```python
from build123d import *

# Parameters (mm, degrees)
CROQUIS1_W              = 8
CROQUIS1_H              = 15
SALIENTE_EXTRUIR6_DEPTH = 1.1
SALIENTE_EXTRUIR7_DEPTH = 2


with BuildPart() as part:
    # Croquis1 → Saliente-Extruir6 (new body)
    with BuildSketch(Plane.XY):
        Rectangle(CROQUIS1_W, CROQUIS1_H)
    extrude(amount=SALIENTE_EXTRUIR6_DEPTH)

    # Croquis8 → Saliente-Extruir7 (add, symmetric)
    with BuildSketch(Plane(origin=(0, 0, 0), x_dir=(0, 0, -1), z_dir=(1, 0, 0))):
        with BuildLine():
            Line((0, 7), (0, 5))
            ThreePointArc((0, 5), (5, 0), (0, -5))
            Line((0, -5), (0, -7))
            ThreePointArc((0, -7), (7, 0), (0, 7))
        make_face()
    extrude(amount=SALIENTE_EXTRUIR7_DEPTH, both=True)


solid = part.part
```
CAD build for the part. Positions are in the model's coordinates, mm. A direction names the side the tool comes from. Round coordinates to 2 decimals unless told otherwise and drop trailing zeros. Order: outer loops, then holes, each group sorted by start corner. A loop starts at its lowest first (then second) coordinate and runs counter-clockwise, first axis right, second up. Notation, with made-up numbers: (48.5, 8.25) -> (80.5, 8.25) arc R22 ccw to (80.5, 24.25) -> close; hole circle Ø8 at (31.25, -24). An arc over 180 degrees is marked (long way). One line per question, with ' | ' between items.
Q1. Slice it at C-C (z = -3.25). Write the cut outline in (x, y), then the cut area to 3 significant figures.
Completed:
outline: (-2, -6.2) -> (2, -6.2) -> (2, -3.8) -> (-2, -3.8) -> close; (-2, 3.8) -> (2, 3.8) -> (2, 6.2) -> (-2, 6.2) -> close | area: 19.2 mm^2
Q2. Which spindle directions (+Z, -Z, +X, -X, +Y, -Y) get a long thin tool onto all of the face, cutting with end or side? Do faces 4 (the flat face through (-2, 2, -5)), 5 (the flat face through (-4, -0.1, 0.5)), 6 (the flat face through (-0.1, -7.5, 0.5)), 7 (the cylindrical face through (0, 0, -5)), 8 (the flat face through (2, 2, -5)). Say none if no direction does.
Completed:
face 4: -Z, -X, +Y, -Y | face 5: +Z, -Z, -X, +Y, -Y | face 6: +Z, -Z, +X, -X, -Y | face 7: +X, -X | face 8: -Z, +X, +Y, -Y
Q3. Two-plate mould, pull along Z, no slides. Class faces 1 (the flat face through (0, 0, 1.1)), 2 (the cylindrical face through (0, 0, -7)), 3 (the flat face through (0, 0, 0)): released by +Z, released by -Z, zero draft, split by the parting line, or undercut.
Completed:
face 1: released by +Z | face 2: released by -Z | face 3: undercut
Q4. Probe probe 1 along Z at (x, y) = (0, 0); probe 2 along X at (y, z) = (1.5, -5); probe 3 along Y at (x, z) = (1.5, -0.75). List the from-to ranges inside material, lowest first.
Completed:
probe 1: z = -7 to -5, 0 to 1.1 | probe 2: x = -2 to 2 | probe 3: y = -6.96 to -4.94, 4.94 to 6.96
Q5. Drop flat-ended pins along their axis: pin 1 (1.5 mm diameter, centred on x = 1.5, z = -5, fed in from -Y); pin 2 (1.5 mm diameter, centred on y = 2, z = -4, fed in from +X); pin 3 (4 mm diameter, centred on x = -1.5, y = 3.5, fed in from -Z). Give the stop position or say it passes through.
Completed:
pin 1: stops at y = -5.56 | pin 2: stops at x = 2 | pin 3: stops at z = -6.84
Q6. Slice it at A-A (x = 0). Write the cut outline in (y, z), then the cut area to 3 significant figures.
Completed:
outline: (-7.5, 0) -> (-7, 0) arc R7 ccw to (7, 0) -> (7.5, 0) -> (7.5, 1.1) -> (-7.5, 1.1) -> close; hole (-5, 0) arc R5 ccw to (5, 0) -> close | area: 54.2 mm^2
Q7. Slice it at B-B (y = 0). Write the cut outline in (x, z), then the cut area to 3 significant figures.
Completed:
outline: (-4, 0) -> (4, 0) -> (4, 1.1) -> (-4, 1.1) -> close; (-2, -7) -> (2, -7) -> (2, -5) -> (-2, -5) -> close | area: 16.8 mm^2
Q8. Slice it at D-D (y = 6.25). Write the cut outline in (x, z).
Completed:
outline: (-4, 0) -> (-2, 0) -> (-2, -3.15) -> (2, -3.15) -> (2, 0) -> (4, 0) -> (4, 1.1) -> (-4, 1.1) -> close
